from build123d import *

# Parameters (mm, degrees)
ESBO_O1_W                = 250
ESBO_O1_H                = 430
RESSALTO_EXTRUS_O1_DEPTH = 15
REVOLU_O1_ANGLE          = 180


with BuildPart() as part:
    # Esboço1 → Ressalto-extrusão1 (new body)
    with BuildSketch(Plane(origin=(0, 0, 0), x_dir=(0, 0, -1), z_dir=(1, 0, 0))):
        Rectangle(ESBO_O1_W, ESBO_O1_H)
    extrude(amount=RESSALTO_EXTRUS_O1_DEPTH)

    # Esboço4 → Revolução1 (revolve)
    with BuildSketch(Plane.ZY):
        with BuildLine():
            Line((-25, 0), (25, 0))
            ThreePointArc((25, 0), (0, -25), (-25, 0))
        make_face()
    revolve(axis=Axis((0, 0, -25), (0, 0, -1)), revolution_arc=REVOLU_O1_ANGLE)


solid = part.part
Source: CAD feature listing. Evaluate the final solid. Frame: model axes, mm. Round coordinates to 2 decimals unless told otherwise and drop trailing zeros. Order: outer loops, then holes, each group sorted by start corner. A loop starts at its lowest first (then second) coordinate and runs counter-clockwise, first axis right, second up. Notation, with made-up numbers: (21.25, -28.5) -> (38.25, -28.5) arc R17 ccw to (38.25, -3.5) -> close; hole circle Ø10 at (-1.5, 9). An arc over 180 degrees is marked (long way). Answer as CSV lines item,"result".
Item 1: Pin query (flat end, axial travel): pin 1 Ø10 at (x, z) = (-6, 20) entering from -Y. Return the tip coordinate at first contact, or that it passes through.
A:
pin 1,"y = -19.31"
Item 2: Line query: L1, parallel to X at y = -87, z = 55; L2, parallel to Y at x = -0.5, z = 12.5. Output: solid intervals per line, ascending.
A:
L1,"0 to 15"
L2,"-21.64 to 21.64"
Item 3: Section C-C, the plane z = -89. Return loops of the section in (x, y).
A:
outline,"(0, -215) -> (15, -215) -> (15, 215) -> (0, 215) -> close"
Item 4: Section D-D, the plane z = -13.5. Return loops of the section in (x, y), plus the area to 3 significant figures.
A:
outline,"(0, -215) -> (15, -215) -> (15, 215) -> (0, 215) -> (0, 21.04) arc R21.04 ccw to (0, -21.04) -> close"
area,"7,150 mm²"
Item 5: Section A-A, the plane x = -15. Return loops of the section in (y, z).
A:
outline,"circle Ø40 at (0, 0)"
Item 6: Section B-B, the plane y = -46. Return loops of the section in (x, z), plus the area to 3 significant figures.
A:
outline,"(0, -125) -> (15, -125) -> (15, 125) -> (0, 125) -> close"
area,"3,750 mm²"
